Check sheet for the modelled part. Datum: model origin and axes. Units: mm. A direction names the side the tool comes from. Give positions to 0.01 mm unless a question says otherwise; leave off trailing zeros. Loops run counter-clockwise (first coordinate to the right, second up) from the corner with the lowest first, then second, coordinate; pieces in that order, holes last.
```python
from build123d import *

# Parameters (mm, degrees)
SKETCH_R           = 30
SKETCH_R_2         = 8
PAD_DEPTH          = 10
POCKET_DEPTH       = 6
POLARPATTERN_COUNT = 8
FILLET_R           = 0.8
FILLET001_R        = 1


with BuildPart() as part:
    # Sketch → Pad (new body, symmetric)
    with BuildSketch(Plane.YZ):
        Circle(SKETCH_R)
        Circle(SKETCH_R_2, mode=Mode.SUBTRACT)
    extrude(amount=PAD_DEPTH, both=True)

    # Sketch001 → Pocket (cut, symmetric)
    with BuildSketch(Plane.YZ):
        with BuildLine():
            ThreePointArc((3.987491, 9.170601), (0, 10), (-3.987491, 9.170601))
            Line((-10.153749, 30.346357), (-3.987491, 9.170601))
            ThreePointArc((10.153749, 30.346357), (0, 32), (-10.153749, 30.346357))
            Line((10.153749, 30.346357), (3.987491, 9.170601))
        make_face()
    pocket = extrude(amount=POCKET_DEPTH, both=True, mode=Mode.SUBTRACT)

    # PolarPattern: Pocket ×8 about axis
    polarpattern_axis = Axis((0, 0, 0), (1, 0, 0))
    for i in range(1, POLARPATTERN_COUNT):
        add(pocket.rotate(polarpattern_axis, i * 360 / POLARPATTERN_COUNT), mode=Mode.SUBTRACT)

    # Fillet
    fillet_edges = [part.edges().sort_by_distance(p)[0] for p in [
        (10, -30, 0),
        (-10, -30, 0),
    ]]
    fillet(fillet_edges, radius=FILLET_R)

    # Fillet001
    fillet001_edges = [part.edges().sort_by_distance(p)[0] for p in [
        (-10, -8, 0),
        (10, -8, 0),
    ]]
    fillet(fillet001_edges, radius=FILLET001_R)


solid = part.part
```
(1) Section check A-A on x = 1.5. Give the number of separate pieces and of enclosed holes in the cut face, plus the area to 3 significant figures.
(2) Material ranges on line 1 (X direction, y = 22.5, z = -0.5); line 2 (Z direction, x = 2, y = 0); line 3 (Y direction, x = 3.5, z = 24.5), recorded low to high.
(3) Release check for a two-part mould opening along X. For faces 1 (the face through (10, 6, 7)), 2 (the face through (-0.13, -1.73, -7.81)), 3 (the face through (0.08, -7.05, 19.69)) record: pulls with the +X half, pulls with the -X half, needs draft (parallel to the pull), parting line crosses it, or undercut.
(4) Section check B-B on z = 0. Record the boundary of the cut face in (x, y).
(5) Gauge pin test, flat ends, axial feed: pin 1 Ø5 at (x, z) = (-1.5, 7.5) entering from +Y; pin 2 Ø12 at (x, z) = (1.5, -6.5) entering from -Y; pin 3 Ø10 at (y, z) = (2.5, -2) entering from +X; pin 4 Ø14.5 at (y, z) = (0, 0) entering from +X. Record the tip position at first contact, or that the pin passes through.
(6) Access from +Z, -Z, +X, -X, +Y, -Y to the whole of each face (thin tool, end or side, straight path). Record for faces 4 (the face through (0.08, 7.05, 19.69)), 5 (the face through (0.08, -19.69, -7.05)), 6 (the face through (0.129, 27.712, -11.49)), 7 (the face through (-6, 14, 0)), 8 (the face through (0.08, 19.69, 7.05)).
Computed values:
1. separate pieces: 9
1. enclosed holes: 1
1. area: 410 mm2
2. line 1: x = -10 to -6, 6 to 10
2. line 2: z = -10 to -8, 8 to 10
2. line 3: y = -12.01 to -8.45, 8.45 to 12.01
3. face 1: pulls with the +X half
3. face 2: needs draft
3. face 3: undercut
4. outline: (-10, -29.2) arc R0.8 ccw to (-9.2, -30) - (-6, -30) - (-6, -10) - (6, -10) - (6, -30) - (9.2, -30) arc R0.8 ccw to (10, -29.2) - (10, -9) arc R1 ccw to (9, -8) - (-9, -8) arc R1 ccw to (-10, -9) - close; (-10, 9) arc R1 ccw to (-9, 8) - (9, 8) arc R1 ccw to (10, 9) - (10, 29.2) arc R0.8 ccw to (9.2, 30) - (6, 30) - (6, 10) - (-6, 10) - (-6, 30) - (-9.2, 30) arc R0.8 ccw to (-10, 29.2) - close
5. pin 1: stops at y = 28.42
5. pin 2: stops at y = -29.89
5. pin 3: stops at x = 9.6
5. pin 4: passes through
6. face 4: +Z
6. face 5: -Y
6. face 6: +X, -X
6. face 7: none
6. face 8: +Y
